Verification items for this drawing (mm, ordinates from the low corner). A direction names the side the tool comes from. Round coordinates to 2 decimals unless told otherwise and drop trailing zeros. Write each loop counter-clockwise with the first axis right and the second up, starting at its lowest first coordinate (ties: lowest second). Pieces come first, ordered by that corner, then holes.
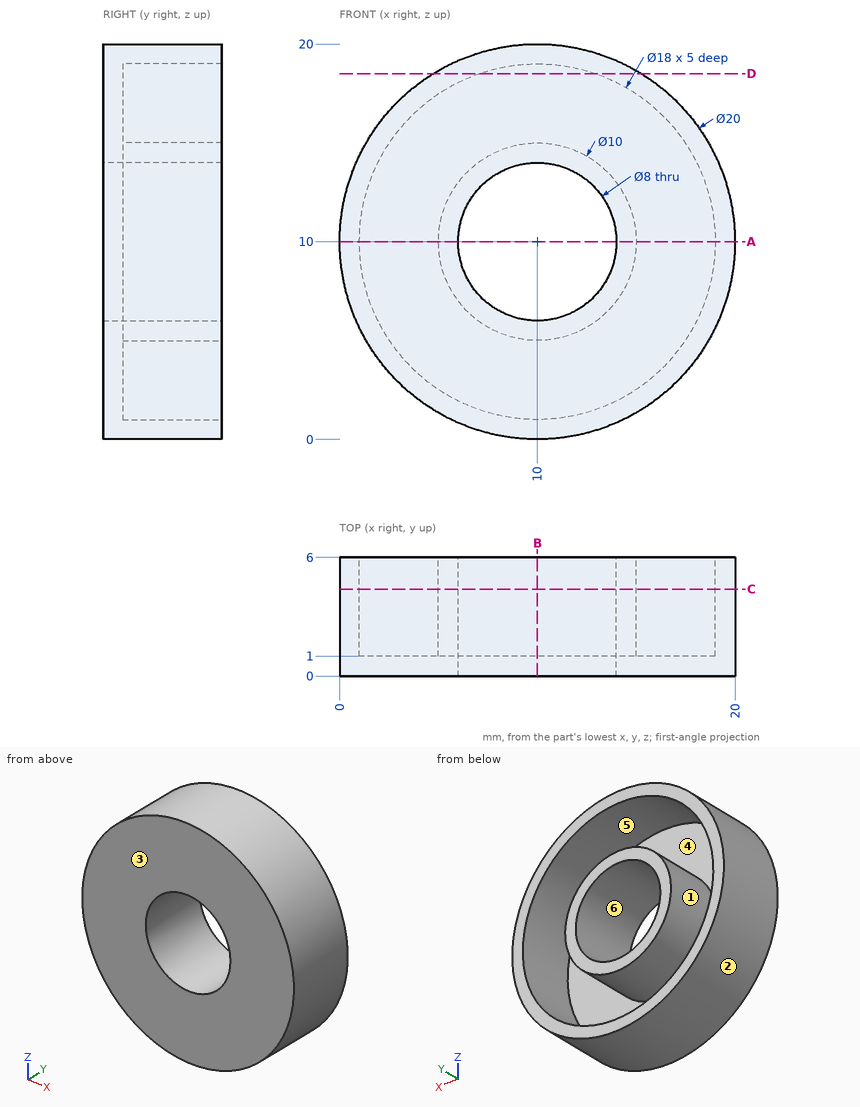
1. Access from +Z, -Z, +X, -X, +Y, -Y to the whole of each face (thin tool, end or side, straight path). Record for the marked faces 5 and 6.
2. Section check D-D (z = 18.5). Record the cut outline in (x, y).
3. Section check A-A (z = 10). Record the cut outline in (x, y), plus the area to 3 significant figures.
4. Release check for a two-part mould opening along X. For the marked faces 1, 2, 3 and 4 record: +X half, -X half, draft (parallel to the pull), parting line (faces both ways), or undercut.
5. Scan lines: line 1 along X through (y, z) = (3.25, 10); line 2 along Y through (x, z) = (4.5, 13.25); line 3 along Z through (x, y) = (9.5, 2.8). Record each from-to range of solid material in increasing order.
6. Depth check by flat-ended pin: pin 1 Ø1.5 at (y, z) = (4.5, 6) entering from +X; pin 2 Ø2 at (x, y) = (6.5, 4) entering from +Z; pin 3 Ø3 at (x, y) = (16.5, 1.5) entering from -Z. Enter the tip coordinate at first touch or a pass-through.
7. Section check C-C (y = 4.4). Record the cut outline in (x, z), plus the area to 3 significant figures.
8. Section check B-B (x = 10). Record the cut outline in (y, z), plus the area to 3 significant figures.
Results below:
1. face 5: +Y
1. face 6: +Y, -Y
2. outline: (4.73, 0) - (15.27, 0) - (15.27, 6) - (12.96, 6) - (12.96, 1) - (7.04, 1) - (7.04, 6) - (4.73, 6) - close
3. outline: (0, 0) - (6, 0) - (6, 6) - (5, 6) - (5, 1) - (1, 1) - (1, 6) - (0, 6) - close; (14, 0) - (20, 0) - (20, 6) - (19, 6) - (19, 1) - (15, 1) - (15, 6) - (14, 6) - close
3. area: 32.0 mm2
4. face 1: undercut
4. face 2: parting line
4. face 3: draft
4. face 4: undercut
5. line 1: x = 0 to 1, 5 to 6, 14 to 15, 19 to 20
5. line 2: y = 0 to 1
5. line 3: z = 0.01 to 1.01, 5.03 to 6.03, 13.97 to 14.97, 18.99 to 19.99
6. pin 1: stops at x = 19.46
6. pin 2: stops at z = 19.68
6. pin 3: stops at z = 1.34
7. outline: circle Ø20 at (10, 10); circle Ø10 at (10, 10); hole circle Ø18 at (10, 10); hole circle Ø8 at (10, 10)
7. area: 88.0 mm2
8. outline: (0, 0) - (6, 0) - (6, 1) - (1, 1) - (1, 5) - (6, 5) - (6, 6) - (0, 6) - close; (0, 14) - (6, 14) - (6, 15) - (1, 15) - (1, 19) - (6, 19) - (6, 20) - (0, 20) - close
8. area: 32.0 mm2
